Solid Edge part; units mm, degrees
sketch "Sketch1" plane through (0, 0, 0) normal (0, -1, 0) x (1, 0, 0)
  line L0 (-17.5, -5) -> (17.5, -5)
  arc A0 (17.5, -5) -> (17.5, 5) centre (17.5, 0) ccw
  line L1 (17.5, 5) -> (-17.5, 5)
  arc A1 (-17.5, -5) -> (-17.5, 5) centre (-17.5, 0) cw
  dimension "D1" = 17.5
  dimension "D2" = 17.5
extrude "Ajout_matière_1" add sketch "Sketch1" against normal blind 3
sketch "Sketch2" plane through (0, 0, 0) normal (0, -1, 0) x (1, 0, 0)
  circle A0 centre (-17.5, 0) radius 1.075
  circle A1 centre (17.5, 0) radius 0.85
extrude "Enlèvement_matière_1" cut sketch "Sketch2" against normal blind 26.6987
properties part number "13" material "MDF 3mm"
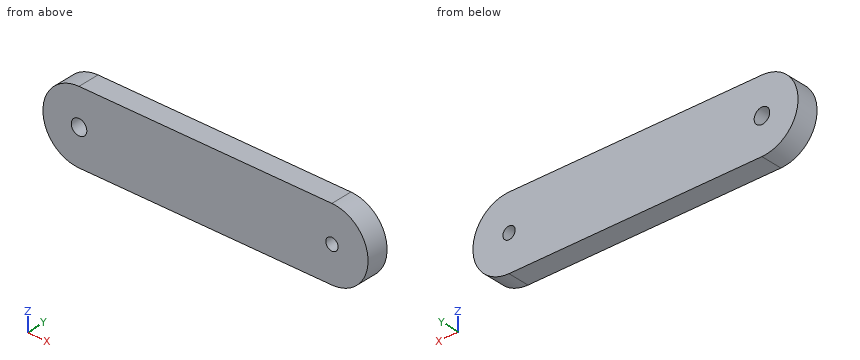
Work out the finished part from the listing and answer in its coordinate system (mm). Give positions to 0.01 mm unless a question says otherwise; leave off trailing zeros. Loops run counter-clockwise (first coordinate to the right, second up) from the corner with the lowest first, then second, coordinate; pieces in that order, holes last. Notation, with made-up numbers: (-22, -35) -> (-5, -35) arc R27 cw to (-5, -16) -> close; hole circle Ø1 at (86, 52). An arc over 180 degrees is marked (long way). Use a Markdown table: item, result. Add a question column.
1. Section A-A on z = 0 is taken. Determine the outline of the cut face in (x, y) (3 decimals).
2. Section C-C on z = -4 is taken. Determine the outline of the cut face in (x, y), and give its area (3 significant figures).
3. Section B-B on y = 2.3 is taken. Determine the outline of the cut face in (x, z) (3 decimals).
4. Find the intervals of material crossed by probe 1 along Z at (x, y) = (-17.5, 1.95) (3 decimals); probe 2 along Z at (x, y) = (17.5, 2.25); probe 3 along X at (y, z) = (2.3, -0.25), in increasing order.
5. Section D-D on x = 19 is taken. Determine the outline of the cut face in (y, z).
Results below:
| question | item | result |
|---|---|---|
| 1 | outline | (-22.5, 0) -> (-18.575, 0) -> (-18.575, 3) -> (-22.5, 3) -> close; (-16.425, 0) -> (16.65, 0) -> (16.65, 3) -> (-16.425, 3) -> close; (18.35, 0) -> (22.5, 0) -> (22.5, 3) -> (18.35, 3) -> close |
| 2 | outline | (-20.5, 0) -> (20.5, 0) -> (20.5, 3) -> (-20.5, 3) -> close |
| 2 | area | 123 mm^2 |
| 3 | outline | (-17.5, -5) -> (17.5, -5) arc R5 ccw to (17.5, 5) -> (-17.5, 5) arc R5 ccw to start; hole circle Ø2.15 at (-17.5, 0); hole circle Ø1.7 at (17.5, 0) |
| 4 | probe 1 | z = -5 to -1.075, 1.075 to 5 |
| 4 | probe 2 | z = -5 to -0.85, 0.85 to 5 |
| 4 | probe 3 | x = -22.49 to -18.55, -16.45 to 16.69, 18.31 to 22.49 |
| 5 | outline | (0, -4.77) -> (3, -4.77) -> (3, 4.77) -> (0, 4.77) -> close |
